from build123d import *

# Parameters (mm, degrees)
F0_R     = 12.7
F1_DEPTH = 127
F3_DEPTH = 12.7


with BuildPart() as f1:
    # F0 (on Front) → F1 (new body)
    with BuildSketch(Plane.XZ):
        Circle(F0_R)
    extrude(amount=F1_DEPTH)

    # F2 (on Top) → F3 (cut, symmetric)
    with BuildSketch(Plane.XY):
        with BuildLine():
            ThreePointArc((6.120889, -8.56995), (-0.59676, -1.8523), (-7.31441, -8.56995))
            Line((-7.31441, -8.56995), (-7.31441, -46.708863))
            ThreePointArc((-7.31441, -46.708863), (-0.59676, -53.426513), (6.120889, -46.708863))
            Line((6.120889, -46.708863), (6.120889, -8.56995))
        make_face()
    extrude(amount=F3_DEPTH, both=True, mode=Mode.SUBTRACT)


solid = f1.part
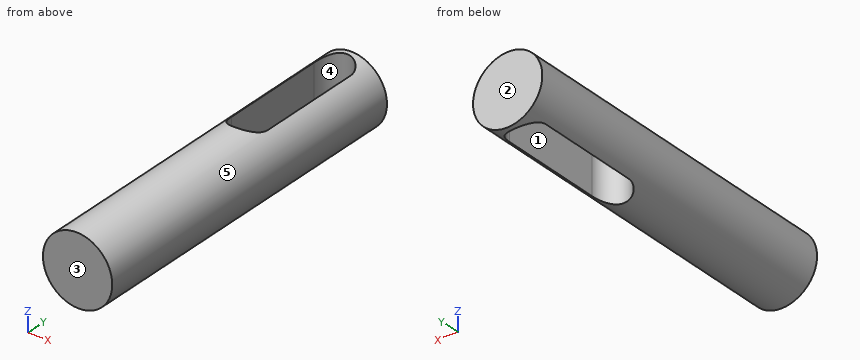
The listing builds one solid part. Answer for the finished solid, in the listing's coordinates (mm). Face numbers are marked on the shaded views. A direction names the side the tool comes from. Give positions to 0.01 mm unless a question says otherwise; leave off trailing zeros. Order: outer loops, then holes, each group sorted by start corner. A loop starts at its lowest first (then second) coordinate and runs counter-clockwise, first axis right, second up. Notation, with made-up numbers: (6, 4) - (44, 4) arc R12 ccw to (44, 20) - close; hole circle Ø9 at (-15, 44.5). An arc over 180 degrees is marked (long way). Use one line per item in the form item = value.
1) The mould has two halves that part along Y. Classify the marked faces 1, 2 and 3: released by +Y, released by -Y, zero draft, split by the parting line, or undercut.
Verdict:
face_1 = undercut
face_2 = released by +Y
face_3 = released by -Y
2) Find section C-C on x = -1.5. Determine the outline of the cut face in (y, z).
Verdict:
outline = (-127, -12.61) - (-53.37, -12.61) - (-53.37, 12.61) - (-127, 12.61) - close; (-1.91, -12.61) - (0, -12.61) - (0, 12.61) - (-1.91, 12.61) - close
3) Each of these flat-tipped pins is pushed along its axis until it touches: pin 1 (6 mm diameter, centred on y = -25, z = -4, fed in from +X); pin 2 (3 mm diameter, centred on y = -48, z = -2, fed in from -X); pin 3 (5 mm diameter, centred on x = -10, y = -29, fed in from +Z). Where does it stop, or does it pass through?
Verdict:
pin_1 = 12.66
pin_2 = -12.69
pin_3 = 10.25
4) Find section B-B on y = -29. Determine the outline of the cut face in (x, z), and give its area (3 significant figures).
Verdict:
outline = (-7.31, -10.38) - (-7.31, 10.38) arc R12.7 ccw to start; (6.12, -11.13) arc R12.7 ccw to (6.12, 11.13) - close
area = 183 mm^2
5) For the marked faces 4 and 5, determine the directions among +Z, -Z, +X, -X, +Y, -Y from which every point of the face is accessible in a straight line to the end or side of a thin tool.
Verdict:
face_4 = +Z, -Z
face_5 = +Y, -Y
6) Consider probe 1 along Y at (x, z) = (-0.25, 6.5); probe 2 along X at (y, z) = (-94.5, 0.75); probe 3 along Y at (x, z) = (2.5, 11.5). Determine where each line is inside the solid, lowest interval first. Write a range as [from, to].
Verdict:
probe_1 = [-127, -53.42], [-1.86, 0]
probe_2 = [-12.68, 12.68]
probe_3 = [-127, -52.67], [-2.61, 0]
7) Find section A-A on z = 0. Determine the outline of the cut face in (x, y).
Verdict:
outline = (-12.7, -127) - (12.7, -127) - (12.7, 0) - (-12.7, 0) - close; hole (-7.31, -46.71) arc R6.72 ccw to (6.12, -46.71) - (6.12, -8.57) arc R6.72 ccw to (-7.31, -8.57) - close
8) Find section D-D on z = -8.25. Determine the outline of the cut face in (x, y), and give its area (3 significant figures).
Verdict:
outline = (-9.66, -127) - (9.66, -127) - (9.66, 0) - (-9.66, 0) - close; hole (-7.31, -46.71) arc R6.72 ccw to (6.12, -46.71) - (6.12, -8.57) arc R6.72 ccw to (-7.31, -8.57) - close
area = 1,800 mm^2
